The figure shows three views and two pictorial views of one solid part (mm, origin at its lowest corner). Answer the questions. A direction names the side the tool comes from. Coordinates: 2 decimals unless noted, no trailing zeros. Write each loop counter-clockwise with the first axis right and the second up, starting at its lowest first coordinate (ties: lowest second). Pieces come first, ordered by that corner, then holes.
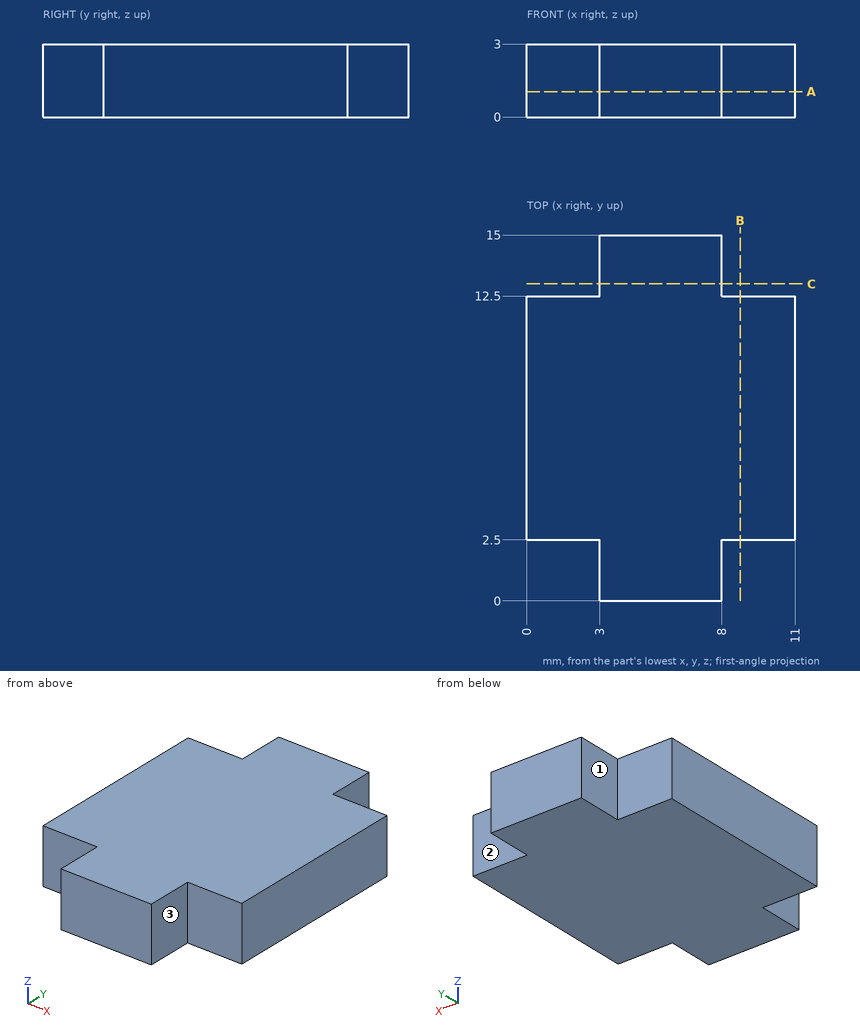
Q1. Which of the six approach directions +Z, -Z, +X, -X, +Y, -Y give full straight-line access (tool end or side, diameter ignored) to the marked faces 1, 2 and 3?
Answers below:
face 1: +Z, -Z, -X, +Y
face 2: +Z, -Z, +X, +Y
face 3: +Z, -Z, +X, -Y
Q2. The part is cut by section B-B, the plane x = 8.75. Write down the section's boundary in (y, z), then the cut area to 3 significant figures.
Answers below:
outline: (2.5, 0) - (12.5, 0) - (12.5, 3) - (2.5, 3) - close
area: 30.0 mm2
Q3. The part is cut by section A-A, the plane z = 1.05. Write down the section's boundary in (x, y), then the cut area to 3 significant figures.
Answers below:
outline: (0, 2.5) - (3, 2.5) - (3, 0) - (8, 0) - (8, 2.5) - (11, 2.5) - (11, 12.5) - (8, 12.5) - (8, 15) - (3, 15) - (3, 12.5) - (0, 12.5) - close
area: 135 mm2
Q4. Given pin 1 (0.9 mm diameter, centred on x = 1, z = 2, fed in from -Y); pin 2 (0.8 mm diameter, centred on y = 14, z = 1, fed in from +X), each flat-ended and moving along its own axis, determine where each tip first touches the part or whether it passes through.
Answers below:
pin 1: stops at y = 2.5
pin 2: stops at x = 8
Q5. The part is cut by section C-C, the plane y = 13. Write down the section's boundary in (x, z).
Answers below:
outline: (3, 0) - (8, 0) - (8, 3) - (3, 3) - close
Q6. Find the intervals of material crossed by probe 1 along Y at (x, z) = (8.75, 0.3); probe 2 along X at (y, z) = (2, 1.5), in increasing order.
Answers below:
probe 1: y = 2.5 to 12.5
probe 2: x = 3 to 8
